```python
from build123d import *

# Parameters (mm, degrees)
F0_W     = 50.8
F0_H     = 31.75
F1_DEPTH = 31.75
F3_DEPTH = 12.7
F5_DEPTH = 25.4
F6_W     = 16.5787817255
F6_H     = 7.9375
F7_DEPTH = 25.4
F8_W     = 16.5787817255
F8_H     = 7.9375
F9_DEPTH = 25.4


with BuildPart() as f1:
    # F0 (on Front) → F1 (new body)
    with BuildSketch(Plane.XZ):
        with Locations((25.4, 15.875)):
            Rectangle(F0_W, F0_H)
    extrude(amount=F1_DEPTH)

    # F2 (on face) → F3 (cut)
    with BuildSketch(Plane.XZ.offset(31.75)):
        Polygon((50.8, 31.75), (17.6424365491, 31.75), (50.8, 0), align=None)
    extrude(amount=-F3_DEPTH, mode=Mode.SUBTRACT)

    # F4 (on face) → F5 (cut)
    with BuildSketch(Plane.XZ.offset(19.05)):
        Polygon((17.6424365491, 31.75), (34.2212182745, 15.875), (34.2212182745, 31.75), align=None)
    extrude(amount=-F5_DEPTH, mode=Mode.SUBTRACT)

    # F6 (on face) → F7 (cut)
    with BuildSketch(Plane.XZ.offset(19.05)):
        with Locations((42.5106091373, 27.78125)):
            Rectangle(F6_W, F6_H)
    extrude(amount=-F7_DEPTH, mode=Mode.SUBTRACT)

    # F8 (on face) → F9 (cut)
    with BuildSketch(Plane.XZ.offset(19.05)):
        with Locations((42.5106091373, 19.84375)):
            Rectangle(F8_W, F8_H)
    extrude(amount=-F9_DEPTH, mode=Mode.SUBTRACT)


solid = f1.part
```
Check sheet for the modelled part. Datum: model origin and axes. Units: mm. A direction names the side the tool comes from. Coordinates: 2 decimals unless noted, no trailing zeros. Write each loop counter-clockwise with the first axis right and the second up, starting at its lowest first coordinate (ties: lowest second). Pieces come first, ordered by that corner, then holes. Notation, with made-up numbers: (23, 80) - (48, 80) arc R31 cw to (48, 116) - close; hole circle Ø10 at (42, 19). An arc over 180 degrees is marked (long way). One line per question, with ' | ' between items.
Item 1: Sectioned sample at A-A on y = -5.5. Record the boundary of the cut face in (x, z) (3 decimals), plus the area to 3 significant figures.
Determined:
outline: (0, 0) - (50.8, 0) - (50.8, 15.875) - (34.221, 15.875) - (17.642, 31.75) - (0, 31.75) - close | area: 1,220 mm2
Item 2: Thickness scan on line 1 (Y direction, x = 46, z = 8.5); line 2 (Z direction, x = 45, y = -16) (3 decimals); line 3 (Z direction, x = 32.5, y = -15.5). Record the ranges inside material, lowest first. Write a range as [from, to].
Determined:
line 1: y = [-19.05, 0] | line 2: z = [0, 15.875] | line 3: z = [0, 17.52]
Item 3: Gauge pin test, flat ends, axial feed: P1, Ø5, axis at x = 35, y = -20.5, coming from the +Z side; P2, Ø4, axis at y = -27, z = 6.5, coming from the +X side; P3, Ø8, axis at y = -14.5, z = 24, coming from the -X side; P4, Ø18, axis at x = 43.5, y = -12, coming from the +Z side (3 decimals). Record the tip position at first contact, or that the pin passes through.
Determined:
P1: stops at z = 17.52 | P2: stops at x = 46.1 | P3: stops at x = 0 | P4: stops at z = 15.875
Item 4: Sectioned sample at D-D on y = -25. Record the boundary of the cut face in (x, z).
Determined:
outline: (0, 0) - (50.8, 0) - (17.64, 31.75) - (0, 31.75) - close
Item 5: Access from +Z, -Z, +X, -X, +Y, -Y to the whole of each face (thin tool, end or side, straight path). Record for faces 1 (the face through (46, -19.05, 12)), 2 (the face through (0, -16, 16)), 3 (the face through (42, -10, 15.875)).
Determined:
face 1: +Z, +X, -Y | face 2: +Z, -Z, -X, +Y, -Y | face 3: +Z, +X, +Y, -Y
Item 6: Sectioned sample at B-B on x = 36.5. Record the boundary of the cut face in (y, z) (3 decimals), plus the area to 3 significant figures.
Determined:
outline: (-31.75, 0) - (0, 0) - (0, 15.875) - (-19.05, 15.875) - (-19.05, 13.693) - (-31.75, 13.693) - close | area: 476 mm2
Item 7: Sectioned sample at C-C on z = 18. Record the boundary of the cut face in (x, y).
Determined:
outline: (0, -31.75) - (32, -31.75) - (32, 0) - (0, 0) - close
